Check sheet for the modelled part. Datum: model origin and axes. Units: mm. Face numbers are marked on the shaded views. A direction names the side the tool comes from. Round coordinates to 2 decimals unless told otherwise and drop trailing zeros. Order: outer loops, then holes, each group sorted by start corner. A loop starts at its lowest first (then second) coordinate and runs counter-clockwise, first axis right, second up.
from build123d import *

# Parameters (mm, degrees)
SKETCH1_W           = 38.1
SKETCH1_H           = 15.24
BOSS_EXTRUDE1_DEPTH = 5.08
SKETCH2_R           = 1.651
CUT_EXTRUDE1_DEPTH  = 119.490202326
SKETCH3_W           = 12.7
SKETCH3_H           = 5.334
BOSS_EXTRUDE2_DEPTH = 30.988
SKETCH6_W           = 45.974
SKETCH6_H           = 5.334
BOSS_EXTRUDE3_DEPTH = 21.59
SKETCH7_R           = 1.778
CUT_EXTRUDE4_DEPTH  = 118.755224526
SKETCH8_R           = 3.937
CUT_EXTRUDE5_DEPTH  = 118.755224526
SKETCH9_W           = 5.334
SKETCH9_H           = 21.59
BOSS_EXTRUDE4_DEPTH = 20
SKETCH10_R          = 1.75
CUT_EXTRUDE6_DEPTH  = 118.755224526
FILLET1_R           = 2
FILLET2_R           = 2


with BuildPart() as part:
    # Sketch1 → Boss-Extrude1 (new body)
    with BuildSketch(Plane(origin=(0, 0, 0), x_dir=(1, 0, 0), z_dir=(0, 1, 0))):
        with Locations((-81.911608108, 54.193229454)):
            Rectangle(SKETCH1_W, SKETCH1_H)
    extrude(amount=-BOSS_EXTRUDE1_DEPTH)

    # Sketch2 → Cut-Extrude1 (cut, through all)
    with BuildSketch(Plane(origin=(0, 0, 0), x_dir=(1, 0, 0), z_dir=(0, 1, 0))):
        with Locations(Location((-94.611608108, 51.907229454, 0), (0, 0, 270))):
            Circle(SKETCH2_R)
        with Locations(Location((-70.481608108, 51.907229454, 0), (0, 0, 270))):
            Circle(SKETCH2_R)
    extrude(amount=-CUT_EXTRUDE1_DEPTH, mode=Mode.SUBTRACT)

    # Sketch3 → Boss-Extrude2 (add)
    with BuildSketch(Plane(origin=(0, 0, 0), x_dir=(1, 0, 0), z_dir=(0, 1, 0))):
        with Locations((-81.911608108, 59.146229454)):
            Rectangle(SKETCH3_W, SKETCH3_H)
    extrude(amount=BOSS_EXTRUDE2_DEPTH)

    # Sketch6 → Boss-Extrude3 (add)
    with BuildSketch(Plane(origin=(0, 30.988, 0), x_dir=(1, 0, 0), z_dir=(0, 1, 0))):
        with Locations((-81.911608108, 59.146229454)):
            Rectangle(SKETCH6_W, SKETCH6_H)
    extrude(amount=BOSS_EXTRUDE3_DEPTH)

    # Sketch7 → Cut-Extrude4 (cut, through all)
    with BuildSketch(Plane.XY.offset(-56.479229454)):
        with Locations((-101.850608108, 33.655)):
            Circle(SKETCH7_R)
        with Locations((-61.972608108, 49.911)):
            Circle(SKETCH7_R)
    extrude(amount=-CUT_EXTRUDE4_DEPTH, mode=Mode.SUBTRACT)

    # Sketch8 → Cut-Extrude5 (cut, through all)
    with BuildSketch(Plane.XY.offset(-56.479229454)):
        with Locations((-81.911608108, 9.906)):
            Circle(SKETCH8_R)
    extrude(amount=-CUT_EXTRUDE5_DEPTH, mode=Mode.SUBTRACT)

    # Sketch9 → Boss-Extrude4 (add)
    with BuildSketch(Plane(origin=(-58.924608108, 0, 0), x_dir=(0, 0, -1), z_dir=(1, 0, 0))):
        with Locations((59.146229454, 41.783)):
            Rectangle(SKETCH9_W, SKETCH9_H)
    extrude(amount=BOSS_EXTRUDE4_DEPTH)

    # Sketch10 → Cut-Extrude6 (cut, through all)
    with BuildSketch(Plane.XY.offset(-56.479229454)):
        with Locations((-46.424608108, 41.783)):
            Circle(SKETCH10_R)
    extrude(amount=-CUT_EXTRUDE6_DEPTH, mode=Mode.SUBTRACT)

    # Fillet1
    fillet1_edges = [part.edges().sort_by_distance(p)[0] for p in [
        (-38.924608108, 30.988, -59.146229454),
        (-38.924608108, 52.578, -59.146229454),
    ]]
    fillet(fillet1_edges, radius=FILLET1_R)

    # Fillet2
    fillet2_edges = [part.edges().sort_by_distance(p)[0] for p in [
        (-104.898608108, 30.988, -59.146229454),
        (-104.898608108, 52.578, -59.146229454),
    ]]
    fillet(fillet2_edges, radius=FILLET2_R)


solid = part.part
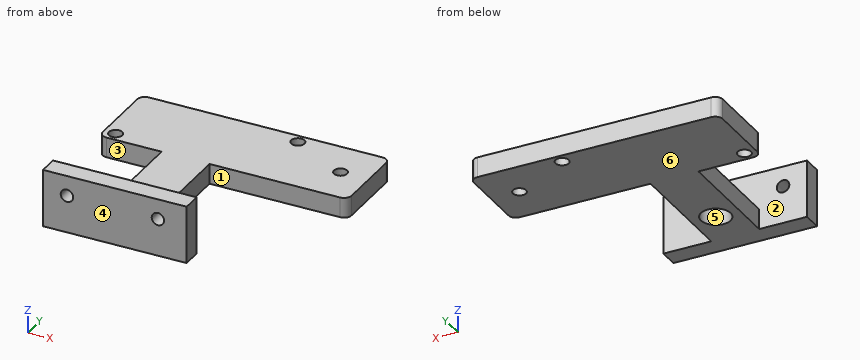
1) Sectioned sample at D-D on y = 8.5. Record the cut outline in (x, z), and give its area (3 significant figures).
2) Sectioned sample at C-C on x = -76.5. Record the cut outline in (y, z), and give its area (3 significant figures).
3) Set-up check for the marked faces 1, 2 and 3: record each of +Z, -Z, +X, -X, +Y, -Y from which the full face is reachable in a straight line by a thin tool's end or side.
4) Sectioned sample at A-A on x = -64.5. Record the cut outline in (y, z).
5) Gauge pin test, flat ends, axial feed: pin 1 (1.5 mm diameter, centred on y = 5.5, z = -55.5, fed in from -X); pin 2 (7.5 mm diameter, centred on x = -89.5, z = -52, fed in from +Y); pin 3 (4.5 mm diameter, centred on y = 20.5, z = -58.5, fed in from +X); pin 4 (5.5 mm diameter, centred on x = -61.97, y = 49.91, fed in from +Z). Record the tip position at first contact, or that the pin passes through.
6) Sectioned sample at B-B on z = -57.75. Record the cut outline in (x, y) (3 decimals), and give its area (3 significant figures).
7) Draft check along Y on the marked faces 4, 5 and 6. Enter one of: pulls with the +Y half, pulls with the -Y half, needs draft (parallel to the pull), parting line crosses it, or undercut.
8) Scan lines: line 1 (Y direction, x = -93, z = -57); line 2 (Z direction, x = -92, y = 41.5); line 3 (Y direction, x = -83, z = -48.5). Record each from-to range of solid material in increasing order.
Values found:
1. outline: (-88.26, -61.81) - (-85.59, -61.81) - (-85.59, -56.48) - (-88.26, -56.48) - close; (-78.23, -61.81) - (-75.56, -61.81) - (-75.56, -56.48) - (-78.23, -56.48) - close
1. area: 28.5 mm2
2. outline: (-5.08, -61.81) - (52.58, -61.81) - (52.58, -56.48) - (0, -56.48) - (0, -46.57) - (-5.08, -46.57) - close
2. area: 358 mm2
3. face 1: +Z, -Z, +X
3. face 2: +Z
3. face 3: +Z, -Z, -X
4. outline: (-5.08, -61.81) - (0, -61.81) - (0, -46.57) - (-5.08, -46.57) - close; (30.99, -61.81) - (52.58, -61.81) - (52.58, -56.48) - (30.99, -56.48) - close
5. pin 1: passes through
5. pin 2: stops at y = 0
5. pin 3: stops at x = -75.56
5. pin 4: stops at z = -56.48
6. outline: (-104.899, 32.988) arc R2 ccw to (-102.899, 30.988) - (-88.262, 30.988) - (-88.262, 0) - (-100.962, 0) - (-100.962, -5.08) - (-62.862, -5.08) - (-62.862, 0) - (-75.562, 0) - (-75.562, 30.988) - (-40.925, 30.988) arc R2 ccw to (-38.925, 32.988) - (-38.925, 50.578) arc R2 ccw to (-40.925, 52.578) - (-102.899, 52.578) arc R2 ccw to (-104.899, 50.578) - close; hole circle Ø3.556 at (-101.851, 33.655); hole circle Ø7.874 at (-81.912, 9.906); hole circle Ø3.556 at (-61.973, 49.911); hole circle Ø3.5 at (-46.425, 41.783)
6. area: 1,930 mm2
7. face 4: pulls with the -Y half
7. face 5: undercut
7. face 6: needs draft
8. line 1: y = -5.08 to 0, 30.99 to 52.58
8. line 2: z = -61.81 to -56.48
8. line 3: y = -5.08 to 0
